Here's how the part is built. I have some questions about the finished solid (model axes, mm). Round coordinates to 2 decimals unless told otherwise and drop trailing zeros. Order: outer loops, then holes, each group sorted by start corner. A loop starts at its lowest first (then second) coordinate and runs counter-clockwise, first axis right, second up. Notation, with made-up numbers: (7.5, -14) -> (30.5, -14) arc R37 ccw to (30.5, 25) -> close; hole circle Ø3 at (-4.5, -36.75). An arc over 180 degrees is marked (long way). Answer in a Markdown table with one row per item.
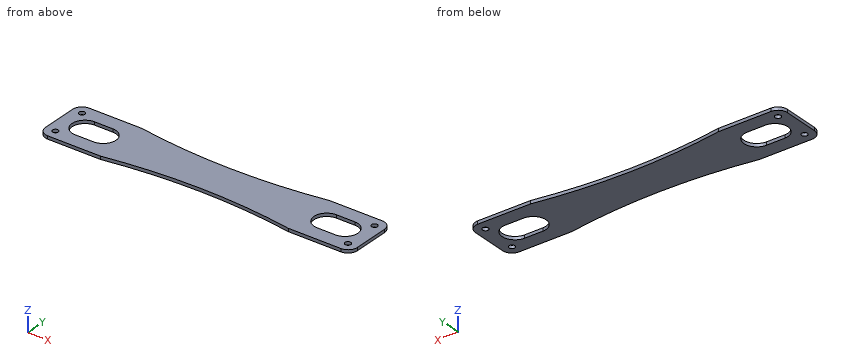
```python
from build123d import *

# Parameters (mm, degrees)
SKETCH_W     = 254
SKETCH_H     = 44.45
SKETCH_R     = 2.3622
PAD_DEPTH    = 2.54
FILLET_R     = 7.62
SKETCH001_R  = 463.55
POCKET_DEPTH = 5.00126


with BuildPart() as part:
    # Sketch → Pad (new body)
    with BuildSketch(Plane.XY):
        with Locations((127, -22.225)):
            Rectangle(SKETCH_W, SKETCH_H)
        with Locations((7.9375, -7.9375)):
            Circle(SKETCH_R, mode=Mode.SUBTRACT)
        with Locations((7.9375, -36.5125)):
            Circle(SKETCH_R, mode=Mode.SUBTRACT)
        with Locations((246.0625, -7.9375)):
            Circle(SKETCH_R, mode=Mode.SUBTRACT)
        with Locations((246.0625, -36.5125)):
            Circle(SKETCH_R, mode=Mode.SUBTRACT)
        with BuildLine():
            ThreePointArc((36.0299, -32.639), (46.4439, -22.225), (36.0299, -11.811))
            Line((36.0299, -11.811), (21.129625, -11.811))
            ThreePointArc((21.129625, -11.811), (10.715625, -22.225), (21.129625, -32.639))
            Line((36.0299, -32.639), (21.129625, -32.639))
        make_face(mode=Mode.SUBTRACT)
        with BuildLine():
            ThreePointArc((232.870375, -32.639), (243.284375, -22.225), (232.870375, -11.811))
            Line((232.870375, -11.811), (217.9701, -11.811))
            ThreePointArc((217.9701, -11.811), (207.5561, -22.225), (217.9701, -32.639))
            Line((232.870375, -32.639), (217.9701, -32.639))
        make_face(mode=Mode.SUBTRACT)
    extrude(amount=PAD_DEPTH)

    # Fillet
    fillet_edges = [part.edges().sort_by_distance(p)[0] for p in [
        (0, -44.45, 1.27),
        (0, 0, 1.27),
        (254, -44.45, 1.27),
        (254, 0, 1.27),
    ]]
    fillet(fillet_edges, radius=FILLET_R)

    # Sketch001 → Pocket (cut)
    with BuildSketch(Plane.XY):
        with Locations((127, -501.65)):
            Circle(SKETCH001_R)
        with Locations((127, 457.2)):
            Circle(SKETCH001_R)
    extrude(amount=POCKET_DEPTH, mode=Mode.SUBTRACT)


solid = part.part
```
1. Suppose I cut it at A-A on x = 220.5. Write out the boundary of the cut face in (y, z), then the cut area to 3 significant figures.
Numbers:
| item | result |
|---|---|
| outline | (-44.45, 0) -> (-32.64, 0) -> (-32.64, 2.54) -> (-44.45, 2.54) -> close; (-11.81, 0) -> (0, 0) -> (0, 2.54) -> (-11.81, 2.54) -> close |
| area | 60.0 mm2 |
2. Suppose I cut it at B-B on y = -41. Write out the boundary of the cut face in (x, z).
Numbers:
| item | result |
|---|---|
| outline | (1.24, 0) -> (75.23, 0) -> (75.23, 2.54) -> (1.24, 2.54) -> close; (178.77, 0) -> (252.76, 0) -> (252.76, 2.54) -> (178.77, 2.54) -> close |
3. Suppose I cut it at D-D on x = 127. Write out the boundary of the cut face in (y, z), then the cut area to 3 significant figures.
Numbers:
| item | result |
|---|---|
| outline | (-38.1, 0) -> (-6.35, 0) -> (-6.35, 2.54) -> (-38.1, 2.54) -> close |
| area | 80.6 mm2 |
4. Please list where these lines run through material, in increasing order: line 1 along X through (y, z) = (-37, 2.35); line 2 along Y through (x, z) = (219, 1.2); line 3 along X through (y, z) = (-38, 1.7).
Numbers:
| item | result |
|---|---|
| line 1 | x = 0 to 5.63, 10.25 to 243.75, 248.37 to 254 |
| line 2 | y = -44.45 to -32.64, -11.81 to 0 |
| line 3 | x = 0.09 to 6.1, 9.77 to 244.23, 247.9 to 253.91 |
5. Suppose I cut it at C-C on z = 1.5. State how many separate pieces and enclosed holes the cut face has, then the cut area to 3 significant figures.
Numbers:
| item | result |
|---|---|
| separate pieces | 1 |
| enclosed holes | 6 |
| area | 8,570 mm2 |
